Verification items for the finished model (mm, model axes). A direction names the side the tool comes from. Coordinates: 2 decimals unless noted, no trailing zeros. Loops run counter-clockwise (first coordinate to the right, second up) from the corner with the lowest first, then second, coordinate; pieces in that order, holes last. Notation, with made-up numbers: (67.5, -34.75) -> (89.5, -34.75) arc R19 ccw to (89.5, -2.75) -> close; hole circle Ø2 at (22, -27). An arc over 180 degrees is marked (long way). Write item = value, one per line.
```python
from build123d import *

# Parameters (mm, degrees)
SKETCH1_W           = 762
SKETCH1_H           = 762
BOSS_EXTRUDE1_DEPTH = 101.6
SKETCH3_W           = 222.25
SKETCH3_H           = 222.25
CUT_EXTRUDE1_DEPTH  = 102.6
BOSS_EXTRUDE2_DEPTH = 50.8
SKETCH5_R           = 6.35
CUT_EXTRUDE2_DEPTH  = 618.31286648
CIRPATTERN1_COUNT   = 4


with BuildPart() as part:
    # Sketch1 → Boss-Extrude1 (new body)
    with BuildSketch(Plane(origin=(0, 0, 0), x_dir=(1, 0, 0), z_dir=(0, 1, 0))):
        Rectangle(SKETCH1_W, SKETCH1_H)
    extrude(amount=BOSS_EXTRUDE1_DEPTH)

    # Sketch3 → Cut-Extrude1 (cut, through all)
    with BuildSketch(Plane(origin=(0, 101.6, 0), x_dir=(1, 0, 0), z_dir=(0, 1, 0))):
        Rectangle(SKETCH3_W, SKETCH3_H)
    extrude(amount=-CUT_EXTRUDE1_DEPTH, mode=Mode.SUBTRACT)

    # Sketch4 → Boss-Extrude2 (add)
    with BuildSketch(Plane(origin=(0, 101.6, 0), x_dir=(1, 0, 0), z_dir=(0, 1, 0))):
        Polygon((141.785512242, 216.876715762), (123.825, 234.837228004), (159.746024484, 270.758252488), (177.706536726, 252.797740246), align=None)
        Polygon((216.876715762, 141.785512242), (252.797740246, 177.706536726), (270.758252488, 159.746024484), (234.837228004, 123.825), align=None)
    boss_extrude2 = extrude(amount=BOSS_EXTRUDE2_DEPTH)

    # Sketch5 → Cut-Extrude2 (cut, through all)
    with BuildSketch(Plane(origin=(55.506114002, 0, 55.506114002), x_dir=(0.707106781, 0, -0.707106781), z_dir=(0.707106781, 0, 0.707106781))):
        with Locations((279.012493577, 127)):
            Circle(SKETCH5_R)
    cut_extrude2 = extrude(amount=-CUT_EXTRUDE2_DEPTH, mode=Mode.SUBTRACT)

    # CirPattern1: Boss-Extrude2, Cut-Extrude2 ×4 about axis
    cirpattern1_axis = Axis((0, 0, 0), (0, 1, 0))
    for i in range(1, CIRPATTERN1_COUNT):
        add(boss_extrude2.rotate(cirpattern1_axis, i * 360 / CIRPATTERN1_COUNT))
        add(cut_extrude2.rotate(cirpattern1_axis, i * 360 / CIRPATTERN1_COUNT), mode=Mode.SUBTRACT)


solid = part.part
```
1) Release check for a two-part mould opening along Z. For faces 4 (the face through (261.904, 126.644, 168.601)), 5 (the face through (-168.852, 126.644, -261.652)), 6 (the face through (246.357, 132.354, -153.054)) record: pulls with the +Z half, pulls with the -Z half, needs draft (parallel to the pull), parting line crosses it, or undercut.
Ans:
face_4 = pulls with the +Z half
face_5 = pulls with the -Z half
face_6 = undercut
2) Sectioned sample at A-A, the plane x = 94.5. Record the cut outline in (y, z) (3 decimals), plus the area to 3 significant figures.
Ans:
outline = (0, -381) -> (101.6, -381) -> (101.6, -111.125) -> (0, -111.125) -> close; (0, 111.125) -> (101.6, 111.125) -> (101.6, 381) -> (0, 381) -> close
area = 54,800 mm2
3) Sectioned sample at D-D, the plane y = 142.5. Count the separate pieces of the cut face and the enclosed holes in it, plus the area to 3 significant figures.
Ans:
separate_pieces = 8
enclosed_holes = 0
area = 10,300 mm2
4) Tool access check on faces 1 (the face through (111.125, 52, 2)), 2 (the face through (257.04, 132.29, -146.03)), 3 (the face through (-225.73, 126.64, -132.93)). Record the directions out of +Z, -Z, +X, -X, +Y, -Y that give a thin tool (end or side, any length) a straight path to the whole face; none if there is none.
Ans:
face_1 = +Y, -Y
face_2 = +X, +Y
face_3 = +Y
5) Material ranges on line 1 (X direction, y = 28, z = 58) (3 decimals); line 2 (Z direction, x = -246, y = 132), recorded low to high.
Ans:
line_1 = -381 to -111.125, 111.125 to 381
line_2 = -170.91 to -154.12, -143.05 to -134.99, 134.99 to 143.05, 154.12 to 170.91
6) Sectioned sample at C-C, the plane z = -27.5. Record the cut outline in (x, y) (3 decimals), plus the area to 3 significant figures.
Ans:
outline = (-381, 0) -> (-111.125, 0) -> (-111.125, 101.6) -> (-381, 101.6) -> close; (111.125, 0) -> (381, 0) -> (381, 101.6) -> (111.125, 101.6) -> close
area = 54,800 mm2
7) Sectioned sample at B-B, the plane y = 19. Record the cut outline in (x, z) (3 decimals), plus the area to 3 significant figures.
Ans:
outline = (-381, -381) -> (381, -381) -> (381, 381) -> (-381, 381) -> close; hole (-111.125, -111.125) -> (111.125, -111.125) -> (111.125, 111.125) -> (-111.125, 111.125) -> close
area = 531,000 mm2
8) Depth check by flat-ended pin: pin 1 Ø5 at (x, z) = (-242.5, -92) entering from +Y. Enter the tip coordinate at first touch or a pass-through.
Ans:
pin_1 = 101.6
